Geometry check sheet. Reference: the model listing, model coordinates, mm. A direction names the side the tool comes from. Round coordinates to 2 decimals unless told otherwise and drop trailing zeros. Write each loop counter-clockwise with the first axis right and the second up, starting at its lowest first coordinate (ties: lowest second). Pieces come first, ordered by that corner, then holes. Notation, with made-up numbers: (39.25, 27) -> (72.25, 27) arc R19 cw to (72.25, 64) -> close; hole circle Ø9 at (60.25, 81.25). An arc over 180 degrees is marked (long way). Use a Markdown table: item, result.
```python
from build123d import *

# Parameters (mm, degrees)
ESQUISSE1_W             = 15
ESQUISSE1_H             = 11
BOSS_EXTRU_1_DEPTH      = 5
ESQUISSE2_R             = 3
BOSS_EXTRU_2_DEPTH      = 20
ENL_V_MAT_EXTRU_1_DEPTH = 10


with BuildPart() as part:
    # Esquisse1 → Boss.-Extru.1 (new body)
    with BuildSketch(Plane.XY):
        Rectangle(ESQUISSE1_W, ESQUISSE1_H)
    extrude(amount=BOSS_EXTRU_1_DEPTH)

    # Esquisse2 → Boss.-Extru.2 (add)
    with BuildSketch(Plane.XY.offset(5)):
        Circle(ESQUISSE2_R)
    extrude(amount=BOSS_EXTRU_2_DEPTH)

    # Esquisse3 → Enlèv. mat.-Extru.1 (cut)
    with BuildSketch(Plane.XY.offset(25)):
        with BuildLine():
            Line((-2.5, -1.658312395), (2.5, -1.658312395))
            ThreePointArc((2.5, -1.658312395), (0, -3), (-2.5, -1.658312395))
        make_face()
    extrude(amount=-ENL_V_MAT_EXTRU_1_DEPTH, mode=Mode.SUBTRACT)


solid = part.part
```
(1) Section check B-B on y = 0. Record the cut outline in (x, z).
A:
| item | result |
|---|---|
| outline | (-7.5, 0) -> (7.5, 0) -> (7.5, 5) -> (3, 5) -> (3, 25) -> (-3, 25) -> (-3, 5) -> (-7.5, 5) -> close |
(2) Section check C-C on z = 9. Record the cut outline in (x, y).
A:
| item | result |
|---|---|
| outline | circle Ø6 at (0, 0) |
(3) Access from +Z, -Z, +X, -X, +Y, -Y to the whole of each face (thin tool, end or side, straight path). Record for faces 1 (the face through (0, 3, 15)), 2 (the face through (0, -1.658, 20)), 3 (the face through (-7.5, 0, 2)).
A:
| item | result |
|---|---|
| face 1 | +Z |
| face 2 | +Z, +X, -X, -Y |
| face 3 | +Z, -Z, -X, +Y, -Y |
(4) Section check A-A on x = 0. Record the cut outline in (y, z).
A:
| item | result |
|---|---|
| outline | (-5.5, 0) -> (5.5, 0) -> (5.5, 5) -> (3, 5) -> (3, 25) -> (-1.66, 25) -> (-1.66, 15) -> (-3, 15) -> (-3, 5) -> (-5.5, 5) -> close |
(5) Section check D-D on x = 5.75. Record the cut outline in (y, z).
A:
| item | result |
|---|---|
| outline | (-5.5, 0) -> (5.5, 0) -> (5.5, 5) -> (-5.5, 5) -> close |
(6) Thickness scan on line 1 (Z direction, x = -6, y = 4); line 2 (X direction, y = -0.25, z = 14); line 3 (X direction, y = -2, z = 6.5). Record the ranges inside material, lowest first.
A:
| item | result |
|---|---|
| line 1 | z = 0 to 5 |
| line 2 | x = -2.99 to 2.99 |
| line 3 | x = -2.24 to 2.24 |
(7) Gauge pin test, flat ends, axial feed: pin 1 Ø3.5 at (x, y) = (3.5, 0) entering from +Z; pin 2 Ø2.5 at (x, z) = (0, 22.5) entering from -Y; pin 3 Ø8 at (x, z) = (2, 13.5) entering from -Y; pin 4 Ø1.5 at (x, z) = (-6, 6) entering from +Y. Record the tip position at first contact, or that the pin passes through.
A:
| item | result |
|---|---|
| pin 1 | stops at z = 25 |
| pin 2 | stops at y = -1.66 |
| pin 3 | stops at y = -3 |
| pin 4 | passes through |
